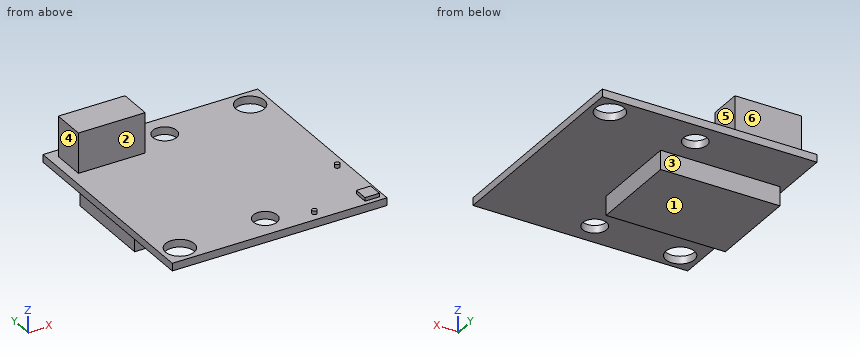
```python
from build123d import *

# Parameters (mm, degrees)
F0_W     = 45
F0_H     = 45
F0_R     = 3
F0_R_2   = 2.5
F1_DEPTH = 1.6
F2_W     = 3
F2_H     = 3
F2_R     = 0.5
F3_DEPTH = 0.75
F4_W     = 25
F4_H     = 19
F5_DEPTH = 4
F6_W     = 14
F6_H     = 7
F7_DEPTH = 8.4


with BuildPart() as f1:
    # F0 (on Top) → F1 (new body)
    with BuildSketch(Plane.XY):
        Rectangle(F0_W, F0_H)
        with Locations((-18.5, -18.5)):
            Circle(F0_R, mode=Mode.SUBTRACT)
        with Locations((0, -17.5)):
            Circle(F0_R_2, mode=Mode.SUBTRACT)
        with Locations((0, 17.5)):
            Circle(F0_R_2, mode=Mode.SUBTRACT)
        with Locations((18.5, 18.5)):
            Circle(F0_R, mode=Mode.SUBTRACT)
    extrude(amount=F1_DEPTH)

    # F2 (on face) → F3 (join)
    with BuildSketch(Plane.XY.offset(1.6)):
        with Locations((20, -20)):
            Rectangle(F2_W, F2_H)
        with Locations((20.5, -8.5)):
            Circle(F2_R)
        with Locations((8.5, -20.5)):
            Circle(F2_R)
    extrude(amount=F3_DEPTH)

    # F4 (on face) → F5 (join)
    with BuildSketch(Plane(origin=(0, 0, 0), x_dir=(1, 0, 0), z_dir=(0, 0, -1))):
        with Locations((-8.769828, -2.14642)):
            Rectangle(F4_W, F4_H)
    extrude(amount=F5_DEPTH)

    # F6 (on face) → F7 (join)
    with BuildSketch(Plane.XY.offset(1.6)):
        with Locations((-13.5, 17)):
            Rectangle(F6_W, F6_H)
    extrude(amount=F7_DEPTH)


solid = f1.part
```
Model file for the job. Use its own axes, mm. Face numbers are marked on the shaded views. A direction names the side the tool comes from. Round coordinates to 2 decimals unless told otherwise and drop trailing zeros. Write each loop counter-clockwise with the first axis right and the second up, starting at its lowest first coordinate (ties: lowest second). Pieces come first, ordered by that corner, then holes. Notation, with made-up numbers: (32.5, -25) -> (48.5, -25) arc R28 cw to (48.5, -4) -> close; hole circle Ø6 at (82.25, 48). An arc over 180 degrees is marked (long way). Answer as CSV lines item,"result".
1. Drill centre lines: line 1 (Y direction, x = 0, z = 1); line 2 (Z direction, x = -16.5, y = 10.5); line 3 (Z direction, x = 12, y = -5.5). Where is each one in solid material? Low to high.
Resolved:
line 1,"-22.5 to -20, -15 to 15, 20 to 22.5"
line 2,"-4 to 1.6"
line 3,"0 to 1.6"
2. Slice it at B-B, the plane y = -17.5. List the corners of the cut face in (x, z).
Resolved:
outline,"(-22.5, 0) -> (-21.33, 0) -> (-21.33, 1.6) -> (-22.5, 1.6) -> close; (-15.67, 0) -> (-2.5, 0) -> (-2.5, 1.6) -> (-15.67, 1.6) -> close; (2.5, 0) -> (22.5, 0) -> (22.5, 1.6) -> (2.5, 1.6) -> close"
3. Pin check, flat tips, straight feed: pin 1 Ø2.5 at (x, z) = (-14.5, 7) entering from +Y; pin 2 Ø4.5 at (y, z) = (1.5, -1.5) entering from +X; pin 3 Ø6.5 at (x, y) = (0, 17.5) entering from -Z; pin 4 Ø0.8 at (x, y) = (20.5, -8.5) entering from +Z. Stop position of each tip, or through.
Resolved:
pin 1,"y = 20.5"
pin 2,"x = 22.5"
pin 3,"z = 0"
pin 4,"z = 2.35"
4. Mould opens along X. For the marked faces 4, 5 and 6 say: +X half, -X half, draft (parallel to the pull), parting line (faces both ways), or undercut.
Resolved:
face 4,"-X half"
face 5,"+X half"
face 6,"draft"
5. Tool access for the marked faces 1, 2 and 3: list every direction of +Z, -Z, +X, -X, +Y, -Y with a clear straight run to the whole face (end or side of a thin tool).
Resolved:
face 1,"-Z, +X, -X, +Y, -Y"
face 2,"+Z, +X, -X, -Y"
face 3,"-Z, +X, -X, +Y"
6. Slice it at D-D, the plane z = 5.75. List the corners of the cut face in (x, y), plus the area to 3 significant figures.
Resolved:
outline,"(-20.5, 13.5) -> (-6.5, 13.5) -> (-6.5, 20.5) -> (-20.5, 20.5) -> close"
area,"98.0 mm²"
7. Slice it at C-C, the plane x = 11. List the corners of the cut face in (y, z), plus the area to 3 significant figures.
Resolved:
outline,"(-22.5, 0) -> (22.5, 0) -> (22.5, 1.6) -> (-22.5, 1.6) -> close"
area,"72.0 mm²"
8. Slice it at A-A, the plane y = 7. List the corners of the cut face in (x, z).
Resolved:
outline,"(-22.5, 0) -> (-21.27, 0) -> (-21.27, -4) -> (3.73, -4) -> (3.73, 0) -> (22.5, 0) -> (22.5, 1.6) -> (-22.5, 1.6) -> close"
